Model file for the job. Use its own axes, mm. Coordinates: 2 decimals unless noted, no trailing zeros. Write each loop counter-clockwise with the first axis right and the second up, starting at its lowest first coordinate (ties: lowest second). Pieces come first, ordered by that corner, then holes. Notation, with made-up numbers: M 83.5,45 L 111.5,45 A34 ccw 111.5,83 Z; hole C -1,-33 d2. An arc over 180 degrees is marked long. Use CSV: the item, a comma, the result in double quotes. Start each with the question number.
from build123d import *

# Parameters (mm, degrees)
F0_W     = 140
F0_H     = 140
F1_DEPTH = 3
F3_D     = 6.8
F3_DEPTH = 10
F4_R     = 5
F6_D     = 62
F6_DEPTH = 10


with BuildPart() as f1:
    # F0 (on Front) → F1 (new body)
    with BuildSketch(Plane.XZ):
        with Locations((-1706.19823, -1509.163168)):
            Rectangle(F0_W, F0_H)
    extrude(amount=F1_DEPTH)

    # F3
    with Locations(Plane.XZ.offset(3)):
        with Locations((-1766.19823, -1449.163168), (-1646.19823, -1449.163168), (-1646.19823, -1569.163168), (-1766.19823, -1569.163168)):
            Hole(F3_D / 2, depth=F3_DEPTH)

    # F4
    f4_edges = [f1.edges().sort_by_distance(p)[0] for p in [
        (-1636.19823, -1.5, -1439.163168),
        (-1636.19823, -1.5, -1579.163168),
        (-1776.19823, -1.5, -1439.163168),
        (-1776.19823, -1.5, -1579.163168),
    ]]
    fillet(f4_edges, radius=F4_R)

    # F6
    with Locations(Plane.XZ.offset(3)):
        with Locations((-1706.19823, -1509.163168)):
            Hole(F6_D / 2, depth=F6_DEPTH)


solid = f1.part
1) Band-saw the part on A-A on x = -1727.5. List the corners of the cut face in (y, z).
2) Band-saw the part on D-D on x = -1648. List the corners of the cut face in (y, z), then the cut area to 3 significant figures.
3) Drop flat-ended pins along their axis: P1, Ø5.5, axis at x = -1646.2, z = -1449.16, coming from the -Y side; P2, Ø9, axis at x = -1766.2, z = -1569.16, coming from the +Y side. Give the stop position or say it passes through.
4) Wall check: L1, parallel to X at y = -1.25, z = -1571.5; L2, parallel to Z at x = -1705, y = -1.2; L3, parallel to Z at x = -1764, y = -2.6. Give the ranges that are in metal, low to high. Write a range as [from, to].
5) Band-saw the part on C-C on y = -1. List the corners of the cut face in (x, z).
6) Band-saw the part on B-B on z = -1516. List the corners of the cut face in (x, y), then the cut area to 3 significant figures.
7) Two-plate mould, pull along X, no slides. Class faces 1 (the face through (-1707, -1, -1579.163)), 2 (the face through (-1769.44, -1.48, -1568.14)), 3 (the face through (-1637.7, -1.52, -1440.59)): pulls with the +X half, pulls with the -X half, needs draft (parallel to the pull), parting line crosses it, or undercut.
Findings below:
1,outline,"M -3,-1579.16 L 0,-1579.16 L 0,-1531.69 L -3,-1531.69 Z; M -3,-1486.64 L 0,-1486.64 L 0,-1439.16 L -3,-1439.16 Z"
2,outline,"M -3,-1579.16 L 0,-1579.16 L 0,-1572.05 L -3,-1572.05 Z; M -3,-1566.28 L 0,-1566.28 L 0,-1452.05 L -3,-1452.05 Z; M -3,-1446.28 L 0,-1446.28 L 0,-1439.16 L -3,-1439.16 Z"
2,area,"385 mm2"
3,P1,"passes through"
3,P2,"stops at y = 0"
4,L1,"x = [-1776.2, -1768.67], [-1763.73, -1648.67], [-1643.73, -1636.2]"
4,L2,"z = [-1579.16, -1540.14], [-1478.19, -1439.16]"
4,L3,"z = [-1579.16, -1571.76], [-1566.57, -1451.76], [-1446.57, -1439.16]"
5,outline,"M -1776.2,-1574.16 A5 ccw -1771.2,-1579.16 L -1641.2,-1579.16 A5 ccw -1636.2,-1574.16 L -1636.2,-1444.16 A5 ccw -1641.2,-1439.16 L -1771.2,-1439.16 A5 ccw -1776.2,-1444.16 Z; hole C -1766.2,-1569.16 d6.8; hole C -1766.2,-1449.16 d6.8; hole C -1706.2,-1509.16 d62; hole C -1646.2,-1569.16 d6.8; hole C -1646.2,-1449.16 d6.8"
6,outline,"M -1776.2,-3 L -1736.43,-3 L -1736.43,0 L -1776.2,0 Z; M -1675.96,-3 L -1636.2,-3 L -1636.2,0 L -1675.96,0 Z"
6,area,"239 mm2"
7,face 1,"needs draft"
7,face 2,"undercut"
7,face 3,"pulls with the +X half"
